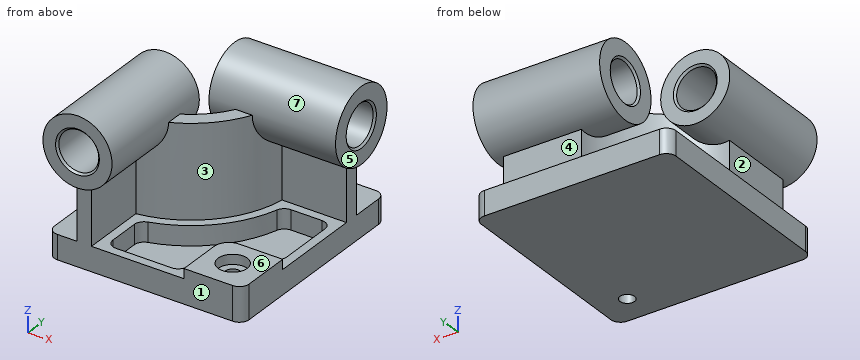
from build123d import *

# Parameters (mm, degrees)
F0_W      = 200
F0_H      = 213
F1_DEPTH  = 25
F3_DEPTH  = 95
F5_DEPTH  = 10
F6_R      = 15
F7_DEPTH  = 10
F8_R      = 7.5
F9_DEPTH  = 25.001
F11_DEPTH = 20
F13_R     = 35.5
F14_DEPTH = 130
F15_R     = 20.5
F16_DEPTH = 223.001
F18_R     = 38.3333333333
F19_DEPTH = 130
F20_R     = 20.5
F21_DEPTH = 210.001
F22_R     = 10
F23_SIZE2 = 2
F23_SIZE  = 2


with BuildPart() as f1:
    # F0 (on Top) → F1 (new body)
    with BuildSketch(Plane.XY):
        with Locations((100, 106.5)):
            Rectangle(F0_W, F0_H)
    extrude(amount=F1_DEPTH)

    # F2 (on face) → F3 (join)
    with BuildSketch(Plane.XY.offset(25)):
        with BuildLine():
            Line((30, 80), (30, 0))
            Line((30, 0), (45, 0))
            Line((45, 0), (45, 66.0769515459))
            ThreePointArc((45, 66.0769515459), (104.2462120246, 95.7537879754), (133.9230484541, 155))
            Line((133.9230484541, 155), (200, 155))
            Line((200, 155), (200, 170))
            Line((200, 170), (120, 170))
            ThreePointArc((120, 170), (93.6396103068, 106.3603896932), (30, 80))
        make_face()
    extrude(amount=F3_DEPTH)

    # F4 (on face) → F5 (join)
    with BuildSketch(Plane.XY.offset(25)):
        with BuildLine():
            Line((200, 60), (155, 60))
            ThreePointArc((155, 60), (144.3933982822, 55.6066017178), (140, 45))
            Line((140, 45), (140, 0))
            Line((140, 0), (200, 0))
            Line((200, 0), (200, 60))
        make_face()
    extrude(amount=F5_DEPTH)

    # F6 (on face) → F7 (cut)
    with BuildSketch(Plane.XY.offset(35)):
        with Locations((168.9159870148, 30.6017436087)):
            Circle(F6_R)
    extrude(amount=-F7_DEPTH, mode=Mode.SUBTRACT)

    # F8 (on face) → F9 (cut, through all)
    with BuildSketch(Plane.XY.offset(25)):
        with Locations((168.9159870148, 30.6017436087)):
            Circle(F8_R)
    extrude(amount=-F9_DEPTH, mode=Mode.SUBTRACT)

    # F10 (on face) → F11 (cut)
    with BuildSketch(Plane.XY.offset(25)):
        with BuildLine():
            Line((181, 146), (149.2476414861, 146))
            ThreePointArc((149.2476414861, 146), (143.2234965193, 143.981834214), (139.630896205, 138.7419354839))
            ThreePointArc((139.630896205, 138.7419354839), (110.6101730553, 89.3898269447), (61.2580645161, 60.369103795))
            ThreePointArc((61.2580645161, 60.369103795), (56.018165786, 56.7765034807), (54, 50.7523585139))
            Line((54, 50.7523585139), (54, 19))
            ThreePointArc((54, 19), (56.9289321881, 11.9289321881), (64, 9))
            Line((64, 9), (121, 9))
            ThreePointArc((121, 9), (128.0710678119, 11.9289321881), (131, 19))
            Line((131, 19), (131, 45))
            ThreePointArc((131, 45), (138.0294372515, 61.9705627485), (155, 69))
            Line((155, 69), (181, 69))
            ThreePointArc((181, 69), (188.0710678119, 71.9289321881), (191, 79))
            Line((191, 79), (191, 136))
            ThreePointArc((191, 136), (188.0710678119, 143.0710678119), (181, 146))
        make_face()
    extrude(amount=-F11_DEPTH, mode=Mode.SUBTRACT)

    # F13 (on offset) → F14 (join)
    with BuildSketch(Plane.XZ.offset(10)):
        with Locations((37.5, 120)):
            Circle(F13_R)
    extrude(amount=-F14_DEPTH)

    # F15 (on face) → F16 (cut, through all)
    with BuildSketch(Plane.XZ.offset(10)):
        with Locations((37.5, 120)):
            Circle(F15_R)
    extrude(amount=-F16_DEPTH, mode=Mode.SUBTRACT)

    # F18 (on offset) → F19 (join)
    with BuildSketch(Plane.YZ.offset(210)):
        with Locations((162.5, 120)):
            Circle(F18_R)
    extrude(amount=-F19_DEPTH)

    # F20 (on face) → F21 (cut, through all)
    with BuildSketch(Plane.YZ.offset(210)):
        with Locations((162.5, 120)):
            Circle(F20_R)
    extrude(amount=-F21_DEPTH, mode=Mode.SUBTRACT)

    # F22
    f22_edges = [f1.edges().sort_by_distance(p)[0] for p in [
        (0, 0, 12.5),
        (200, 0, 17.5),
        (200, 213, 12.5),
        (0, 213, 12.5),
    ]]
    fillet(f22_edges, radius=F22_R)

    # F23
    f23_edges = [f1.edges().sort_by_distance(p)[0] for p in [
        (17, -10, 120),
        (210, 142, 120),
        (17, 120, 120),
        (80, 142, 120),
    ]]
    chamfer(f23_edges, length=F23_SIZE, length2=F23_SIZE2)


solid = f1.part
Verification items for the finished model (mm, model axes). Face numbers are marked on the shaded views. A direction names the side the tool comes from. Coordinates: 2 decimals unless noted, no trailing zeros. Order: outer loops, then holes, each group sorted by start corner. A loop starts at its lowest first (then second) coordinate and runs counter-clockwise, first axis right, second up. Notation, with made-up numbers: M 58.5,-37 L 86.5,-37 A18 cw 86.5,-23 Z; hole C 80.25,86.5 d11. An arc over 180 degrees is marked long. Return JSON: item names as keys, results as strings.
1) Cross-section at B-B, the plane x = 37.5. Record the boundary of the cut face in (y, z), and give its area (3 significant figures).
Answer list:
{"outline": "M -10,84.5 L 0,84.5 L 0,0 L 213,0 L 213,25 L 80.31,25 L 80.31,84.5 L 120,84.5 L 120,97.5 L 118,99.5 L -8,99.5 L -10,97.5 Z; M -10,142.5 L -8,140.5 L 118,140.5 L 120,142.5 L 120,155.5 L -10,155.5 Z", "area": "14,000 mm2"}
2) Thickness scan on L1, parallel to Z at x = 37.5, y = 90; L2, parallel to Z at x = 41.5, y = 97; L3, parallel to Z at x = 137, y = 162. Record the ranges inside material, lowest first. Write a range as [from, to].
Answer list:
{"L1": "[0, 25], [84.5, 99.5], [140.5, 155.5]", "L2": "[0, 25], [84.73, 99.89], [140.11, 155.27]", "L3": "[0, 99.51], [140.49, 158.33]"}
3) Cross-section at D-D, the plane y = 162.5. Record the boundary of the cut face in (x, z).
Answer list:
{"outline": "M 0,0 L 200,0 L 200,81.67 L 210,81.67 L 210,97.5 L 208,99.5 L 82,99.5 L 80,97.5 L 80,81.67 L 119.69,81.67 L 119.69,25 L 0,25 Z; M 80,142.5 L 82,140.5 L 208,140.5 L 210,142.5 L 210,158.33 L 80,158.33 Z"}
4) Gauge pin test, flat ends, axial feed: pin 1 (6 mm diameter, centred on x = 166.5, z = 13, fed in from -Y); pin 2 (23 mm diameter, centred on y = 171, z = 118, fed in from -X); pin 3 (12 mm diameter, centred on x = 134.5, y = 83.5, fed in from +Z); pin 4 (8 mm diameter, centred on x = 23.5, y = 97.5, fed in from +Z). Record the tip position at first contact, or that the pin passes through.
Answer list:
{"pin 1": "y = 0", "pin 2": "through", "pin 3": "z = 5", "pin 4": "z = 154.06"}
5) Access from +Z, -Z, +X, -X, +Y, -Y to the whole of each face (thin tool, end or side, straight path). Record for the marked faces 1, 2, 3 and 4.
Answer list:
{"face 1": "-Z, +X, -X, -Y", "face 2": "-X, +Y, -Y", "face 3": "+X, -Y", "face 4": "+X, -X, +Y"}
6) Release check for a two-part mould opening along Z. For the marked faces 5, 6 and 7 record: +Z half, -Z half, draft (parallel to the pull), parting line (faces both ways), or undercut.
Answer list:
{"face 5": "draft", "face 6": "+Z half", "face 7": "undercut"}
7) Cross-section at A-A, the plane z = 69.5. Record the boundary of the cut face in (x, y), and give its area (3 significant figures).
Answer list:
{"outline": "M 30,0 L 45,0 L 45,66.08 A105 ccw 133.92,155 L 200,155 L 200,170 L 120,170 A90 cw 30,80 Z", "area": "4,260 mm2"}
8) Cross-section at C-C, the plane x = 143. Record the boundary of the cut face in (y, z).
Answer list:
{"outline": "M 0,0 L 213,0 L 213,25 L 170,25 L 170,82.41 A38.33 ccw long 155,82.41 L 155,25 L 143.81,25 L 143.81,5 L 65.78,5 L 65.78,25 L 54,25 L 54,35 L 0,35 Z; hole C 162.5,120 d41"}
